Could you check a few things on this drawing? It's one solid part, dimensions in mm from its lowest x, y, z. A direction names the side the tool comes from. Coordinates: 2 decimals unless noted, no trailing zeros. Order: outer loops, then holes, each group sorted by start corner. A loop starts at its lowest first (then second) coordinate and runs counter-clockwise, first axis right, second up. Notation, with made-up numbers: (74.5, -13.75) -> (121.5, -13.75) arc R24 ccw to (121.5, 13.25) -> close; hole circle Ø9 at (31.5, -16.5). An arc over 180 degrees is marked (long way). Answer as CSV lines item,"result".
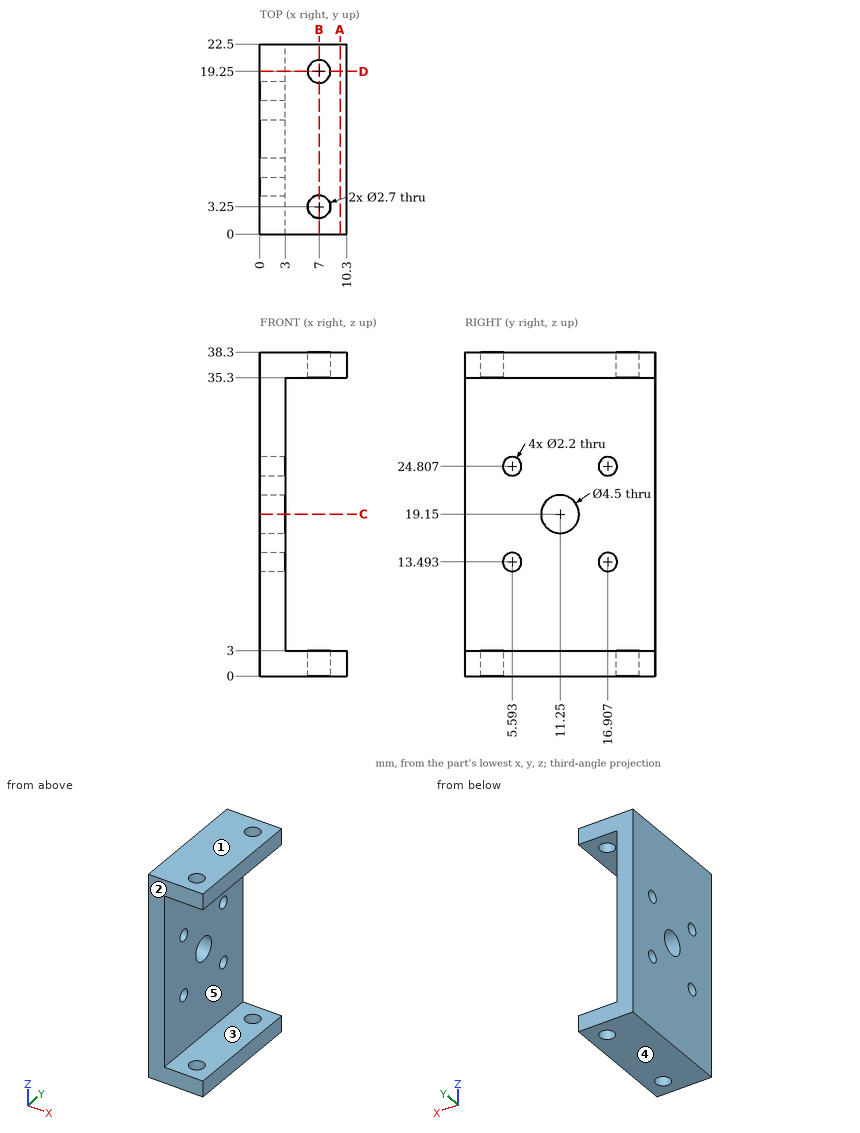
Q1. For P1, Ø2.5, axis at x = 7, y = 3.25, coming from the +Z side (3 decimals); P2, Ø5, axis at x = 3.5, y = 12, coming from the -Z side; P3, Ø7, axis at y = 6, z = 24.5, coming from the +X side, each with a flat end and sliding along its axis, tell me the tip position at first contact or that it passes through.
Solution:
P1,"through"
P2,"z = 0"
P3,"x = 3"
Q2. Imagine slicing it at C-C (z = 19.15). List the corners of the cut face in (x, y) for me.
Solution:
outline,"(0, 0) -> (3, 0) -> (3, 9) -> (0, 9) -> close; (0, 13.5) -> (3, 13.5) -> (3, 22.5) -> (0, 22.5) -> close"
Q3. Which directions (+Z, -Z, +X, -X, +Y, -Y) give clear straight access to the entire face, cutting with the end or side of a thin tool? Please do the marked faces 4 and 5.
Solution:
face 4,"-Z, +X, -X, +Y, -Y"
face 5,"+X, +Y, -Y"
Q4. Imagine slicing it at B-B (x = 7). List the corners of the cut face in (y, z) for me.
Solution:
outline,"(0, 0) -> (1.9, 0) -> (1.9, 3) -> (0, 3) -> close; (0, 35.3) -> (1.9, 35.3) -> (1.9, 38.3) -> (0, 38.3) -> close; (4.6, 0) -> (17.9, 0) -> (17.9, 3) -> (4.6, 3) -> close; (4.6, 35.3) -> (17.9, 35.3) -> (17.9, 38.3) -> (4.6, 38.3) -> close; (20.6, 0) -> (22.5, 0) -> (22.5, 3) -> (20.6, 3) -> close; (20.6, 35.3) -> (22.5, 35.3) -> (22.5, 38.3) -> (20.6, 38.3) -> close"
Q5. We'd pull the mould along Z, two halves only. Please class the marked faces 1, 2 and 3: pulls with the +Z half, pulls with the -Z half, needs draft (parallel to the pull), parting line crosses it, or undercut.
Solution:
face 1,"pulls with the +Z half"
face 2,"needs draft"
face 3,"undercut"
Q6. If I drill on line 1 (Y direction, x = 7, z = 2.2); line 2 (Z direction, x = 5, y = 7.75); line 3 (Z direction, x = 2.75, y = 6) (1 decimal), over which ranges is the centre line in solid material (lowest first)?
Solution:
line 1,"0 to 1.9, 4.6 to 17.9, 20.6 to 22.5"
line 2,"0 to 3, 35.3 to 38.3"
line 3,"0 to 12.5, 14.5 to 23.8, 25.8 to 38.3"
Q7. Imagine slicing it at D-D (y = 19.25). List the corners of the cut face in (x, z) for me, and give its area (4 significant figures).
Solution:
outline,"(0, 0) -> (5.65, 0) -> (5.65, 3) -> (3, 3) -> (3, 35.3) -> (5.65, 35.3) -> (5.65, 38.3) -> (0, 38.3) -> close; (8.35, 0) -> (10.3, 0) -> (10.3, 3) -> (8.35, 3) -> close; (8.35, 35.3) -> (10.3, 35.3) -> (10.3, 38.3) -> (8.35, 38.3) -> close"
area,"142.5 mm2"
Q8. Imagine slicing it at A-A (x = 9.5). List the corners of the cut face in (y, z) for me.
Solution:
outline,"(0, 0) -> (22.5, 0) -> (22.5, 3) -> (0, 3) -> close; (0, 35.3) -> (22.5, 35.3) -> (22.5, 38.3) -> (0, 38.3) -> close"
